from build123d import *

# Parameters (mm, degrees)
SKETCH_1_R      = 25
SKETCH_1_R_2    = 1.326040619
SKETCH_1_R_3    = 1.707538373
SKETCH_1_R_4    = 1.989060928
SKETCH_1_R_5    = 1.868114934
EXTRUDE_1_DEPTH = 30
SKETCH_2_R      = 20
EXTRUDE_2_DEPTH = 5
SKETCH_3_R      = 10
EXTRUDE_3_DEPTH = 20


with BuildPart() as part:
    # 草图1 → 凸台-拉伸1 (new body)
    with BuildSketch(Plane(origin=(0, 0, 0), x_dir=(1, 0, 0), z_dir=(0, 1, 0))):
        with Locations(Location((0, 0, 0), (0, 0, 270))):
            Circle(SKETCH_1_R)
        with Locations(Location((0, 3.551894514, 0), (0, 0, 270))):
            Circle(SKETCH_1_R_2, mode=Mode.SUBTRACT)
        with Locations(Location((0, 8.19303668, 0), (0, 0, 270))):
            Circle(SKETCH_1_R_3, mode=Mode.SUBTRACT)
        with Locations(Location((0, 21.453442867, 0), (0, 0, 270))):
            Circle(SKETCH_1_R_4, mode=Mode.SUBTRACT)
        with Locations(Location((0, 14.349653838, 0), (0, 0, 270))):
            Circle(SKETCH_1_R_5, mode=Mode.SUBTRACT)
        with Locations(Location((2.776982954, 2.214570007, 0), (0, 0, 270))):
            Circle(SKETCH_1_R_2, mode=Mode.SUBTRACT)
        with Locations(Location((6.405574013, 5.108274816, 0), (0, 0, 270))):
            Circle(SKETCH_1_R_3, mode=Mode.SUBTRACT)
        with Locations(Location((11.219011133, 8.946862828, 0), (0, 0, 270))):
            Circle(SKETCH_1_R_5, mode=Mode.SUBTRACT)
        with Locations(Location((16.77297704, 13.376002842, 0), (0, 0, 270))):
            Circle(SKETCH_1_R_4, mode=Mode.SUBTRACT)
        with Locations(Location((3.462841103, -0.790370885, 0), (0, 0, 270))):
            Circle(SKETCH_1_R_2, mode=Mode.SUBTRACT)
        with Locations(Location((7.987620145, -1.823122174, 0), (0, 0, 270))):
            Circle(SKETCH_1_R_3, mode=Mode.SUBTRACT)
        with Locations(Location((13.989878057, -3.193098374, 0), (0, 0, 270))):
            Circle(SKETCH_1_R_5, mode=Mode.SUBTRACT)
        with Locations(Location((20.915560263, -4.773840143, 0), (0, 0, 270))):
            Circle(SKETCH_1_R_4, mode=Mode.SUBTRACT)
        with Locations(Location((1.541109273, -3.200146379, 0), (0, 0, 270))):
            Circle(SKETCH_1_R_2, mode=Mode.SUBTRACT)
        with Locations(Location((3.554825389, -7.381670982, 0), (0, 0, 270))):
            Circle(SKETCH_1_R_3, mode=Mode.SUBTRACT)
        with Locations(Location((6.226081462, -12.928591373, 0), (0, 0, 270))):
            Circle(SKETCH_1_R_5, mode=Mode.SUBTRACT)
        with Locations(Location((9.308300008, -19.328884132, 0), (0, 0, 270))):
            Circle(SKETCH_1_R_4, mode=Mode.SUBTRACT)
        with Locations(Location((-1.541109273, -3.200146379, 0), (0, 0, 270))):
            Circle(SKETCH_1_R_2, mode=Mode.SUBTRACT)
        with Locations(Location((-3.554825389, -7.381670982, 0), (0, 0, 270))):
            Circle(SKETCH_1_R_3, mode=Mode.SUBTRACT)
        with Locations(Location((-6.226081462, -12.928591373, 0), (0, 0, 270))):
            Circle(SKETCH_1_R_5, mode=Mode.SUBTRACT)
        with Locations(Location((-9.308300008, -19.328884132, 0), (0, 0, 270))):
            Circle(SKETCH_1_R_4, mode=Mode.SUBTRACT)
        with Locations(Location((-3.462841103, -0.790370885, 0), (0, 0, 270))):
            Circle(SKETCH_1_R_2, mode=Mode.SUBTRACT)
        with Locations(Location((-7.987620145, -1.823122174, 0), (0, 0, 270))):
            Circle(SKETCH_1_R_3, mode=Mode.SUBTRACT)
        with Locations(Location((-13.989878057, -3.193098374, 0), (0, 0, 270))):
            Circle(SKETCH_1_R_5, mode=Mode.SUBTRACT)
        with Locations(Location((-20.915560263, -4.773840143, 0), (0, 0, 270))):
            Circle(SKETCH_1_R_4, mode=Mode.SUBTRACT)
        with Locations(Location((-2.776982954, 2.214570007, 0), (0, 0, 270))):
            Circle(SKETCH_1_R_2, mode=Mode.SUBTRACT)
        with Locations(Location((-6.405574013, 5.108274816, 0), (0, 0, 270))):
            Circle(SKETCH_1_R_3, mode=Mode.SUBTRACT)
        with Locations(Location((-11.219011133, 8.946862828, 0), (0, 0, 270))):
            Circle(SKETCH_1_R_5, mode=Mode.SUBTRACT)
        with Locations(Location((-16.77297704, 13.376002842, 0), (0, 0, 270))):
            Circle(SKETCH_1_R_4, mode=Mode.SUBTRACT)
    extrude(amount=EXTRUDE_1_DEPTH)

    # 草图2 → 凸台-拉伸2 (add)
    with BuildSketch(Plane(origin=(0, 30, 0), x_dir=(1, 0, 0), z_dir=(0, 1, 0))):
        with Locations(Location((0, 0, 0), (0, 0, 86.243341215))):
            Circle(SKETCH_2_R)
    extrude(amount=EXTRUDE_2_DEPTH)

    # 草图3 → 凸台-拉伸3 (add)
    with BuildSketch(Plane(origin=(0, 35, 0), x_dir=(1, 0, 0), z_dir=(0, 1, 0))):
        with Locations(Location((0, 0, 0), (0, 0, 270))):
            Circle(SKETCH_3_R)
    extrude(amount=EXTRUDE_3_DEPTH)


solid = part.part
The model under review builds one solid part; all positions refer to its coordinate system, in mm. Round coordinates to 2 decimals unless told otherwise and drop trailing zeros. Write each loop counter-clockwise with the first axis right and the second up, starting at its lowest first coordinate (ties: lowest second). Pieces come first, ordered by that corner, then holes. Notation, with made-up numbers: M -21,15 L 8,15 A17 ccw 8,22 Z; hole C 2.25,71.5 d8. An arc over 180 degrees is marked long. Use a Markdown table: item, result. Add a question column.
Q1. We need section C-C, the plane y = 51. State the section outline as (x, z) points, plus the area to 3 significant figures.
Q2. Insertion check: pin 1 (2 mm diameter, centred on y = 24.5, z = -16.5, fed in from +X); pin 2 (3 mm diameter, centred on x = -8.5, y = 49, fed in from -Z); pin 3 (5 mm diameter, centred on y = 30, z = 0.5, fed in from -X). Each pin has a flat end and moves straight along its axis. Give the tip position at first contact, or say it passes through.
Q3. To check wall thickness, follow line 1 (X direction, y = 8, z = -10.5); line 2 (Z direction, x = 3.5, y = 17); line 3 (Z direction, x = -15.5, y = 25). State the ranges of each line that lie inside material, in increasing order.
Q4. We need section A-A, the plane y = 12.5. Count the separate pieces of the cut face and the enclosed holes in it, plus the area to 3 significant figures.
Q5. We need section B-B, the plane z = 14. State the section outline as (x, y) points.
Q6. The part is to be moulded in two halves that separate along Z. For faces 1 (the face through (7.509, 14.79, 23.846)), 2 (the face through (-9, 35, -5)), 3 (the face through (1.599, 14.79, 1.875)), say which applies: pulls with the +Z half, pulls with the -Z half, needs draft (parallel to the pull), parting line crosses it, or undercut.
Findings below:
| question | item | result |
|---|---|---|
| 1 | outline | C 0,0 d20 |
| 1 | area | 314 mm² |
| 2 | pin 1 | stops at x = 19.62 |
| 2 | pin 2 | stops at z = -7.14 |
| 2 | pin 3 | stops at x = -25 |
| 3 | line 1 | x = -22.69 to -12.26, -10.18 to 10.18, 12.26 to 22.69 |
| 3 | line 2 | z = -24.75 to -3.33, -1.1 to -0.54, 2.12 to 5.68, 9.09 to 24.75 |
| 3 | line 3 | z = -19.62 to -14.9, -11.85 to 2.09, 4.29 to 19.62 |
| 4 | separate pieces | 1 |
| 4 | enclosed holes | 28 |
| 4 | area | 1,700 mm² |
| 5 | outline | M -20.71,0 L -7.76,0 L -7.76,30 L -4.7,30 L -4.7,0 L 4.7,0 L 4.7,30 L 7.76,30 L 7.76,0 L 20.71,0 L 20.71,30 L 14.28,30 L 14.28,35 L -14.28,35 L -14.28,30 L -20.71,30 Z |
| 6 | face 1 | parting line crosses it |
| 6 | face 2 | needs draft |
| 6 | face 3 | undercut |
